Answer from the drawing. Dimensions are ordinates in mm from the lowest x, y and z of the part. A direction names the side the tool comes from. Coordinates: 2 decimals unless noted, no trailing zeros. Loops run counter-clockwise (first coordinate to the right, second up) from the corner with the lowest first, then second, coordinate; pieces in that order, holes last. Notation, with made-up numbers: M -21,56 L 32,56 A24 ccw 32,79 Z; hole C -38.5,-38 d11. An arc over 180 degrees is marked long. One line per item, written item: value. Start each with the question number.
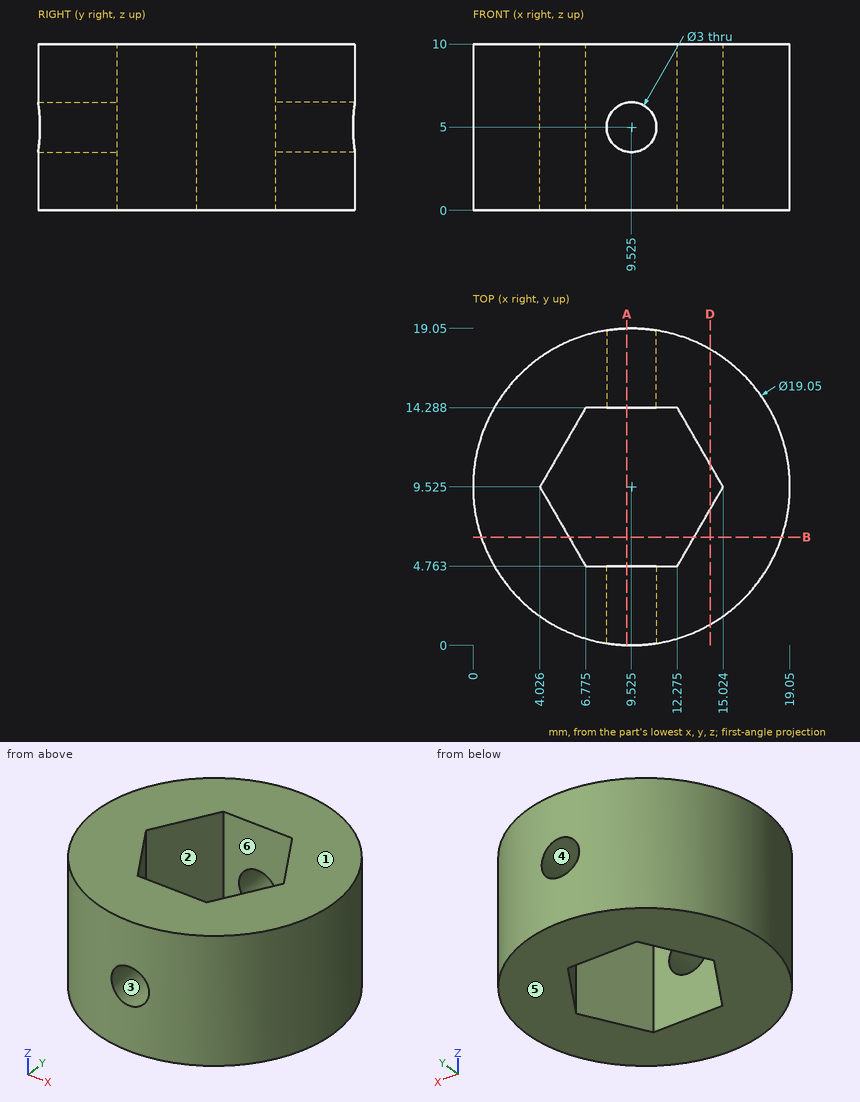
1) Section B-B (y = 6.5) is taken. Determine the outline of the cut face in (x, z).
2) Section D-D (x = 14.25) is taken. Determine the outline of the cut face in (y, z) (1 decimal).
3) Section A-A (x = 9.25) is taken. Determine the outline of the cut face in (y, z) (1 decimal).
4) For a pull along Z with two mould halves and no side action, classify the marked faces 3, 4, 5 and 6 as released by +Z, released by -Z, zero draft, split by the parting line, or undercut.
5) Consider line 1 along Y through (x, z) = (12, 0.75); line 2 along X through (y, z) = (8.5, 5) (1 decimal); line 3 along X through (y, z) = (8, 3.5) (1 decimal). Determine where each line is inside the solid, lowest interval first.
6) Flat-ended cylindrical pins translate along their axes: pin 1 (6 mm diameter, centred on x = 17, z = 7.5, fed in from -Y); pin 2 (1.8 mm diameter, centred on x = 9.525, z = 5, fed in from -Y); pin 3 (3 mm diameter, centred on y = 13.5, z = 7.5, fed in from -X); pin 4 (1.5 mm diameter, centred on y = 4, z = 5, fed in from -X). Find the tip coordinate at first contact, or state that the pin passes through.
7) A tool of negligible diameter and unlimited length cuts with its end or side. For the marked faces 1 and 2, from which of +Z, -Z, +X, -X, +Y, -Y can it reach the whole face along a straight path? Write none if from no direction.
Results found:
1. outline: M 0.49,0 L 5.77,0 L 5.77,10 L 0.49,10 Z; M 13.28,0 L 18.56,0 L 18.56,10 L 13.28,10 Z
2. outline: M 1.3,0 L 8.2,0 L 8.2,10 L 1.3,10 Z; M 10.9,0 L 17.8,0 L 17.8,10 L 10.9,10 Z
3. outline: M 0,0 L 4.8,0 L 4.8,3.5 L 0,3.5 Z; M 0,6.5 L 4.8,6.5 L 4.8,10 L 0,10 Z; M 14.3,0 L 19,0 L 19,3.5 L 14.3,3.5 Z; M 14.3,6.5 L 19,6.5 L 19,10 L 14.3,10 Z
4. face 3: undercut
4. face 4: undercut
4. face 5: released by -Z
4. face 6: zero draft
5. line 1: y = 0.33 to 4.76, 14.29 to 18.72
5. line 2: x = 0.1 to 4.6, 14.4 to 19
5. line 3: x = 0.1 to 4.9, 14.1 to 18.9
6. pin 1: stops at y = 1.12
6. pin 2: passes through
6. pin 3: stops at x = 0.33
6. pin 4: stops at x = 1.28
7. face 1: +Z, +X, -X, +Y, -Y
7. face 2: +Z, -Z
